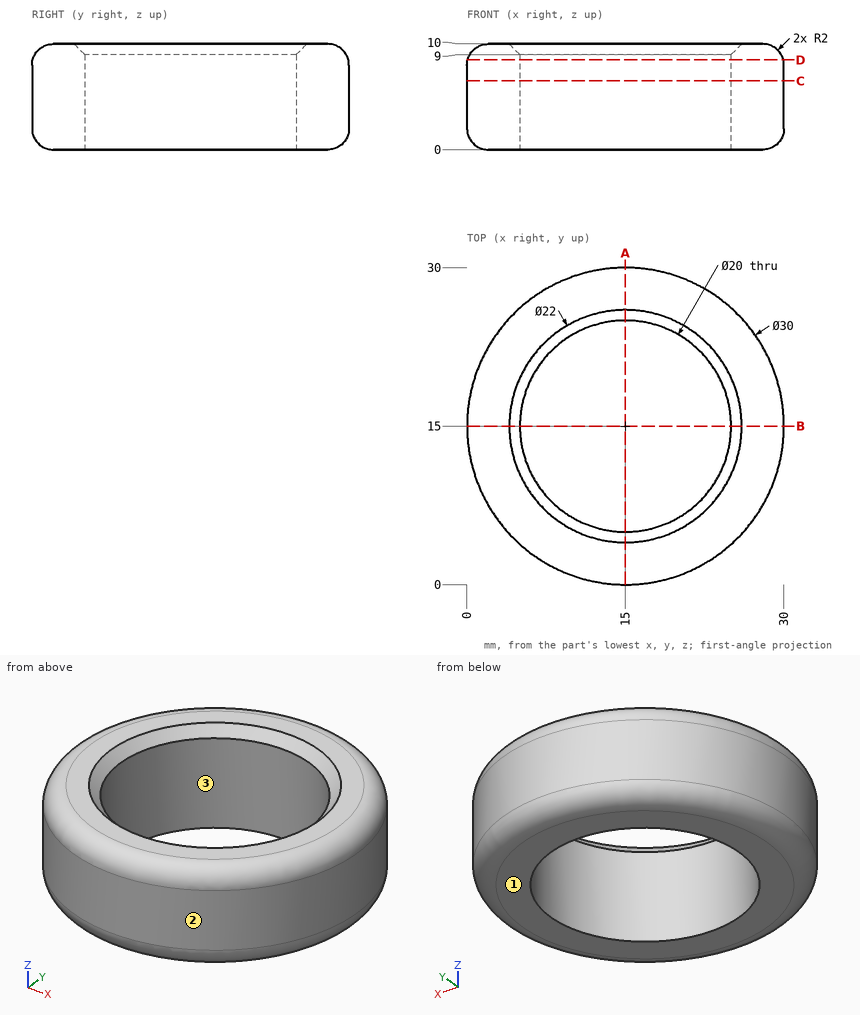
Geometry check sheet. Reference: drawing and pictorial views, mm from the part's lowest x, y, z. Round coordinates to 2 decimals unless told otherwise and drop trailing zeros. Write each loop counter-clockwise with the first axis right and the second up, starting at its lowest first coordinate (ties: lowest second). Pieces come first, ordered by that corner, then holes.
1. Scan lines: L1, parallel to Y at x = 15, z = 6.5; L2, parallel to X at y = 15.75, z = 7.5; L3, parallel to X at y = 14, z = 3.5. Record each from-to range of solid material in increasing order.
2. Gauge pin test, flat ends, axial feed: P1, Ø4, axis at y = 9, z = 5.5, coming from the +X side; P2, Ø10, axis at x = 18.5, y = 3, coming from the -Z side; P3, Ø1.5, axis at y = 17.5, z = 3.5, coming from the +X side; P4, Ø5, axis at x = 22, z = 8, coming from the -Y side. Record the tip position at first contact, or that the pin passes through.
3. Section check A-A on x = 15. Enter the section's corners in (y, z).
4. Section check C-C on z = 6.5. Enter the section's corners in (x, y), plus the area to 3 significant figures.
5. Section check D-D on z = 8.5. Enter the section's corners in (x, y), plus the area to 3 significant figures.
6. Draft check along Y on the marked faces 1, 2 and 3. Enter one of: +Y half, -Y half, draft (parallel to the pull), parting line (faces both ways), or undercut.
Answer:
1. L1: y = 0 to 5, 25 to 30
1. L2: x = 0.02 to 5.03, 24.97 to 29.98
1. L3: x = 0.03 to 5.05, 24.95 to 29.97
2. P1: stops at x = 29.46
2. P2: stops at z = 0
2. P3: stops at x = 29.9
2. P4: stops at y = 0.69
3. outline: (0, 2) arc R2 ccw to (2, 0) - (5, 0) - (5, 9) - (4, 10) - (2, 10) arc R2 ccw to (0, 8) - close; (25, 0) - (28, 0) arc R2 ccw to (30, 2) - (30, 8) arc R2 ccw to (28, 10) - (26, 10) - (25, 9) - close
4. outline: circle Ø30 at (15, 15); hole circle Ø20 at (15, 15)
4. area: 393 mm2
5. outline: circle Ø29.87 at (15, 15); hole circle Ø20 at (15, 15)
5. area: 387 mm2
6. face 1: draft
6. face 2: parting line
6. face 3: undercut
